The model under review builds one solid part; all positions refer to its coordinate system, in mm. A direction names the side the tool comes from. Coordinates: 2 decimals unless noted, no trailing zeros. Loops run counter-clockwise (first coordinate to the right, second up) from the corner with the lowest first, then second, coordinate; pieces in that order, holes last. Notation, with made-up numbers: M 8.25,-2.75 L 37.25,-2.75 A28 cw 37.25,36.25 Z; hole C -14,-12.75 d8. An arc over 180 degrees is marked long. Return JSON: item names as keys, results as strings.
Autodesk Inventor part; units mm, degrees
ref_plane "YZ Plane" through (0, 0, 0) normal (1, 0, 0) x (0, 1, 0)
ref_plane "XZ Plane" through (0, 0, 0) normal (0, 1, 0) x (-1, 0, 0)
ref_plane "XY Plane" through (0, 0, 0) normal (0, 0, 1) x (1, 0, 0)
sketch "Sketch1" plane through (0, 0, 0) normal (0, 1, 0) x (-1, 0, 0)
  line L0 (10.9985, -6.35) -> (0, -12.7)
  line L1 (0, -12.7) -> (-10.9985, -6.35)
  line L2 (-10.9985, -6.35) -> (-10.9985, 6.35)
  line L3 (-10.9985, 6.35) -> (0, 12.7)
  line L4 (0, 12.7) -> (10.9985, 6.35)
  line L5 (10.9985, 6.35) -> (10.9985, -6.35)
  point P0 (0, 0)
  point P1 (0, 0)
  dimension "d0" = 25.4
extrude "Extrusion1" add sketch "Sketch1" along normal blind 10.16
sketch "Sketch2" plane through (0, 10.16, 0) normal (0, 1, 0) x (1, 0, 0)
  circle A0 centre (0, 0) radius 10.9985
extrude "Extrusion2" cut sketch "Sketch2" against normal through all draft 45 keep common part
sketch "Sketch3" plane through (0, 0, 0) normal (0, -1, 0) x (1, 0, 0)
  circle A0 centre (0, 0) radius 6.35
  dimension "d5" = 12.7
extrude "Extrusion3" add sketch "Sketch3" along normal blind 22.86
thread "Thread1"
properties part number "Bolt"
1. Add section A-A on y = 6.5. Give the boundary of the cut face in (x, z), plus the area to 3 significant figures.
Check values:
{"outline": "M -11,-6.35 L 0,-12.7 L 11,-6.35 L 11,6.35 L 0,12.7 L -11,6.35 Z", "area": "419 mm²"}
2. Insertion check: pin 1 Ø12 at (x, y) = (8, -18.5) entering from +Z; pin 2 Ø1 at (y, z) = (0, 7) entering from +X; pin 3 Ø8 at (y, z) = (-7, 7) entering from -X. Each pin has a flat end and moves straight along its axis. Give the tip position at first contact, or say it passes through.
Check values:
{"pin 1": "z = 6.03", "pin 2": "x = 10.74", "pin 3": "x = -5.6"}
3. Machinability: for faces 1 (the face through (-5.58, 5.01, -9.48)), 2 (the face through (5, 0, -5)), which of the approach directions +Z, -Z, +X, -X, +Y, -Y give a long, thin tool a straight path to every point of the face, cutting with its end or side? Answer none if there is none.
Check values:
{"face 1": "-Z, -X, +Y, -Y", "face 2": "-Y"}
4. Add section B-B on y = -21. Give the boundary of the cut face in (x, z).
Check values:
{"outline": "C 0,0 d12.7"}
5. To check wall thickness, follow line 1 (Y direction, x = -8.75, z = 0); line 2 (X direction, y = -3, z = 2.5); line 3 (Z direction, x = -3.75, y = -6.5). State the ranges of each line that lie inside material, in increasing order.
Check values:
{"line 1": "0 to 10.16", "line 2": "-5.84 to 5.84", "line 3": "-5.12 to 5.12"}
